For this review, take the finished solid that the model builds, in its own axes (mm). Face numbers are marked on the shaded views. A direction names the side the tool comes from. Round coordinates to 2 decimals unless told otherwise and drop trailing zeros. Loops run counter-clockwise (first coordinate to the right, second up) from the corner with the lowest first, then second, coordinate; pieces in that order, holes last. Notation, with made-up numbers: (86.25, 10) -> (122.25, 10) arc R20 cw to (122.25, 38) -> close; hole circle Ø5 at (80, 53). An arc over 180 degrees is marked (long way). One line per question, with ' | ' between items. Start each with the question number.
1. Consider section D-D (y = -21.05). Write out the cut boundary in (x, z), and give its area (3 significant figures).
2. For pin 1 Ø2 at (x, y) = (28.15, -2) entering from +Z; pin 2 Ø5 at (y, z) = (-4, 20) entering from -X; pin 3 Ø3 at (x, y) = (46.15, -2) entering from +Z; pin 4 Ø12 at (y, z) = (-11.5, 18.5) entering from +X, all flat-tipped, find the tip position at first contact; note any pin that passes through.
3. Consider section C-C (z = 20). Write out the cut boundary in (x, y), and give its area (3 significant figures).
4. Wall thickness on line 1 along Y through (x, z) = (28.15, 4); line 2 along Z through (x, y) = (20.5, -20.25); line 3 along X through (y, z) = (-20.75, 18.5): over which ranges is each line inside the solid? List them lowest first.
5. Consider section B-B (x = 28.15). Write out the cut boundary in (y, z).
6. Consider section A-A (y = -2). Write out the cut boundary in (x, z).
7. For the marked faces 1 and 2, list the 3-axis set-ups (+Z, -Z, +X, -X, +Y, -Y) from which the entire face can be reached by the end or side of a thin tool; tool diameter is ignored.
```python
from build123d import *

# Parameters (mm, degrees)
SKETCH1_W           = 57.15
SKETCH1_H           = 25
BOSS_EXTRUDE1_DEPTH = 5
SKETCH2_R           = 1.25
SKETCH2_R_2         = 1.27
CUT_EXTRUDE2_DEPTH  = 6
SKETCH5_W           = 10
SKETCH5_H           = 25
BOSS_EXTRUDE3_DEPTH = 20
FILLET1_R           = 10
SKETCH6_R           = 1.7
CUT_EXTRUDE3_DEPTH  = 11


with BuildPart() as part:
    # Sketch1 → Boss-Extrude1 (new body)
    with BuildSketch(Plane.XY):
        with Locations((28.575, -12.5)):
            Rectangle(SKETCH1_W, SKETCH1_H)
    extrude(amount=BOSS_EXTRUDE1_DEPTH)

    # Sketch2 → Cut-Extrude2 (cut, through all)
    with BuildSketch(Plane.XY.offset(5)):
        with Locations((28.15, -2)):
            Circle(SKETCH2_R)
        with Locations((46.15, -2)):
            Circle(SKETCH2_R)
        with Locations((28.15, -21.05)):
            Circle(SKETCH2_R_2)
        with Locations((46.15, -21.05)):
            Circle(SKETCH2_R_2)
    extrude(amount=-CUT_EXTRUDE2_DEPTH, mode=Mode.SUBTRACT)

    # Sketch5 → Boss-Extrude3 (add)
    with BuildSketch(Plane.XY.offset(5)):
        with Locations((5, -12.5)):
            Rectangle(SKETCH5_W, SKETCH5_H)
    extrude(amount=BOSS_EXTRUDE3_DEPTH)

    # Fillet1
    fillet1_edges = [part.edges().sort_by_distance(p)[0] for p in [
        (10, -12.5, 5),
    ]]
    fillet(fillet1_edges, radius=FILLET1_R)

    # Sketch6 → Cut-Extrude3 (cut, through all)
    with BuildSketch(Plane(origin=(10, 0, 0), x_dir=(0, 0, -1), z_dir=(1, 0, 0))):
        with Locations((-20, -21.834919238)):
            Circle(SKETCH6_R)
        with Locations((-20, -5.503108416)):
            Circle(SKETCH6_R)
    extrude(amount=-CUT_EXTRUDE3_DEPTH, mode=Mode.SUBTRACT)


solid = part.part
```
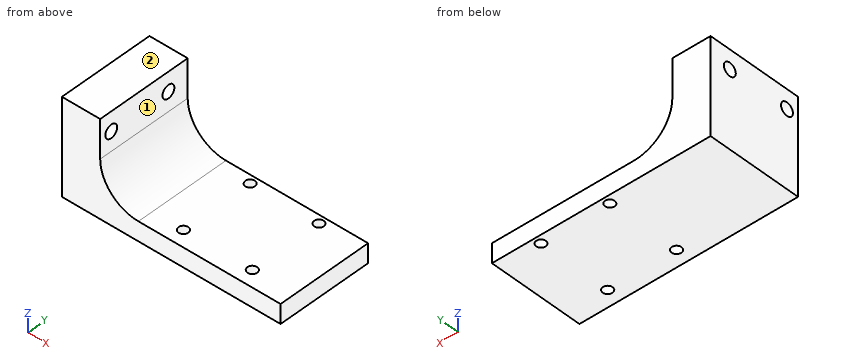
Answer block:
1) outline: (0, 0) -> (26.88, 0) -> (26.88, 5) -> (20, 5) arc R10 cw to (10, 15) -> (10, 18.49) -> (0, 18.49) -> close; (0, 21.51) -> (10, 21.51) -> (10, 25) -> (0, 25) -> close; (29.42, 0) -> (44.88, 0) -> (44.88, 5) -> (29.42, 5) -> close; (47.42, 0) -> (57.15, 0) -> (57.15, 5) -> (47.42, 5) -> close | area: 452 mm2
2) pin 1: passes through | pin 2: stops at x = 0 | pin 3: stops at z = 5 | pin 4: stops at x = 10.32
3) outline: (0, -25) -> (10, -25) -> (10, -23.53) -> (0, -23.53) -> close; (0, -20.13) -> (10, -20.13) -> (10, -7.2) -> (0, -7.2) -> close; (0, -3.8) -> (10, -3.8) -> (10, 0) -> (0, 0) -> close | area: 182 mm2
4) line 1: y = -25 to -22.32, -19.78 to -3.25, -0.75 to 0 | line 2: z = 0 to 5 | line 3: x = 0 to 10
5) outline: (-25, 0) -> (-22.32, 0) -> (-22.32, 5) -> (-25, 5) -> close; (-19.78, 0) -> (-3.25, 0) -> (-3.25, 5) -> (-19.78, 5) -> close; (-0.75, 0) -> (0, 0) -> (0, 5) -> (-0.75, 5) -> close
6) outline: (0, 0) -> (26.9, 0) -> (26.9, 5) -> (20, 5) arc R10 cw to (10, 15) -> (10, 25) -> (0, 25) -> close; (29.4, 0) -> (44.9, 0) -> (44.9, 5) -> (29.4, 5) -> close; (47.4, 0) -> (57.15, 0) -> (57.15, 5) -> (47.4, 5) -> close
7) face 1: +Z, +X, +Y, -Y | face 2: +Z, +X, -X, +Y, -Y
